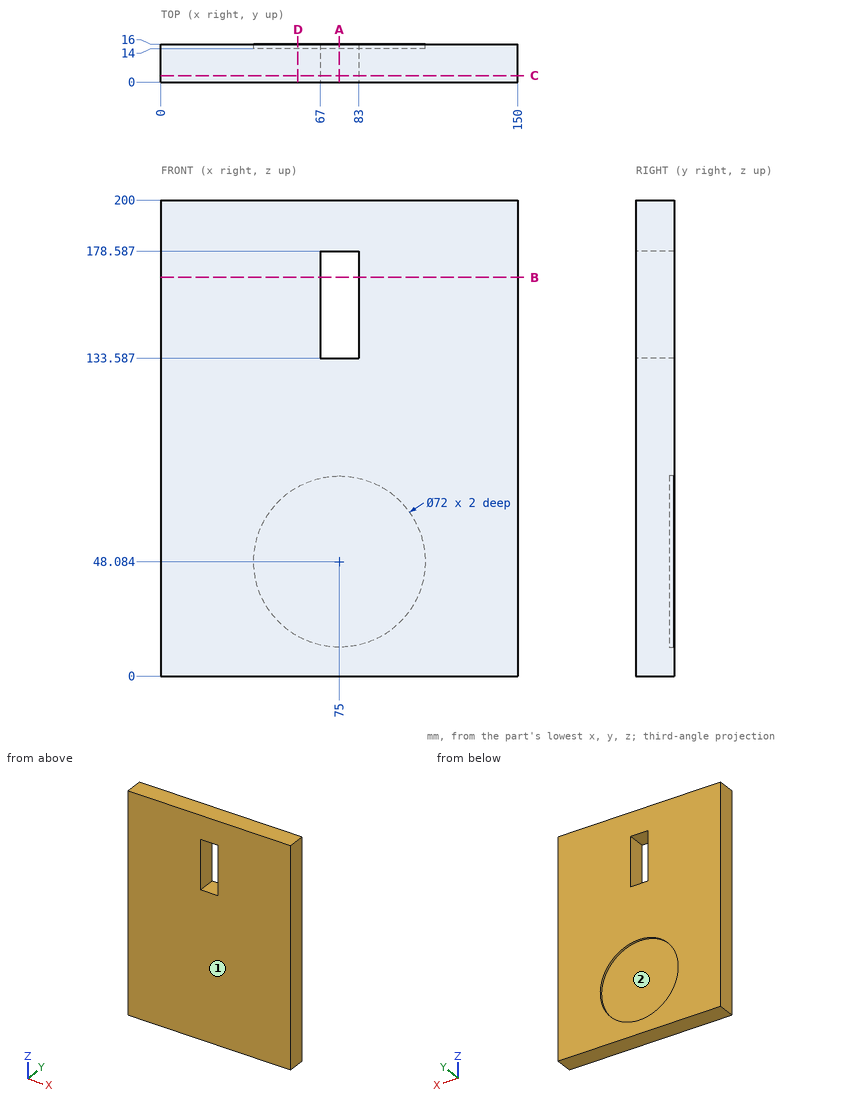
Source: three-view drawing plus pictorial views. Frame: mm from the lowest corner of the part. Give positions to 0.01 mm unless a question says otherwise; leave off trailing zeros. Loops run counter-clockwise (first coordinate to the right, second up) from the corner with the lowest first, then second, coordinate; pieces in that order, holes last. Notation, with made-up numbers: (-9.5, 57.5) -> (9.5, 57.5) arc R21 ccw to (9.5, 78.5) -> close; hole circle Ø1 at (71, 59). An arc over 180 degrees is marked (long way). Put each result on its own line as item: value. Start each with the question number.
1) Cut plane A-A (x = 75). Return loops of the section in (y, z), then the cut area to 3 significant figures.
2) Material intervals for probe 1 along X at (y, z) = (10.25, 140.5); probe 2 along Z at (x, y) = (75, 2); probe 3 along Y at (x, z) = (107, 49), sorted ascending.
3) Cut plane C-C (y = 2.75). Return loops of the section in (x, z).
4) Cut plane B-B (z = 167.5). Return loops of the section in (x, y).
5) Draft query along Z for the marked faces 1 and 2. Return one class per face: released by +Z, released by -Z, zero draft, split by the parting line, or undercut.
6) Cut plane D-D (x = 57.5). Return loops of the section in (y, z).
7) Contact query for a flat-ended pin moving along its axis: P1, Ø2, axis at x = 91, y = 8, coming from the -Z side. Output: stop coordinate, or through.
Results are:
1. outline: (0, 0) -> (16, 0) -> (16, 12.08) -> (14, 12.08) -> (14, 84.08) -> (16, 84.08) -> (16, 133.59) -> (0, 133.59) -> close; (0, 178.59) -> (16, 178.59) -> (16, 200) -> (0, 200) -> close
1. area: 2,340 mm2
2. probe 1: x = 0 to 67, 83 to 150
2. probe 2: z = 0 to 133.59, 178.59 to 200
2. probe 3: y = 0 to 14
3. outline: (0, 0) -> (150, 0) -> (150, 200) -> (0, 200) -> close; hole (67, 133.59) -> (83, 133.59) -> (83, 178.59) -> (67, 178.59) -> close
4. outline: (0, 0) -> (67, 0) -> (67, 16) -> (0, 16) -> close; (83, 0) -> (150, 0) -> (150, 16) -> (83, 16) -> close
5. face 1: zero draft
5. face 2: undercut
6. outline: (0, 0) -> (16, 0) -> (16, 16.62) -> (14, 16.62) -> (14, 79.54) -> (16, 79.54) -> (16, 200) -> (0, 200) -> close
7. P1: stops at z = 0
